Job drawing, mm, ordinate dimensions from the low corner. One solid piece. A direction names the side the tool comes from. Give positions to 0.01 mm unless a question says otherwise; leave off trailing zeros. Order: outer loops, then holes, each group sorted by start corner. A loop starts at its lowest first (then second) coordinate and runs counter-clockwise, first axis right, second up. Notation, with made-up numbers: M 79.5,65 L 100.5,65 A16 cw 100.5,70 Z; hole C -32,-28.75 d9. An arc over 180 degrees is marked long. One line per question, with ' | ' between items.
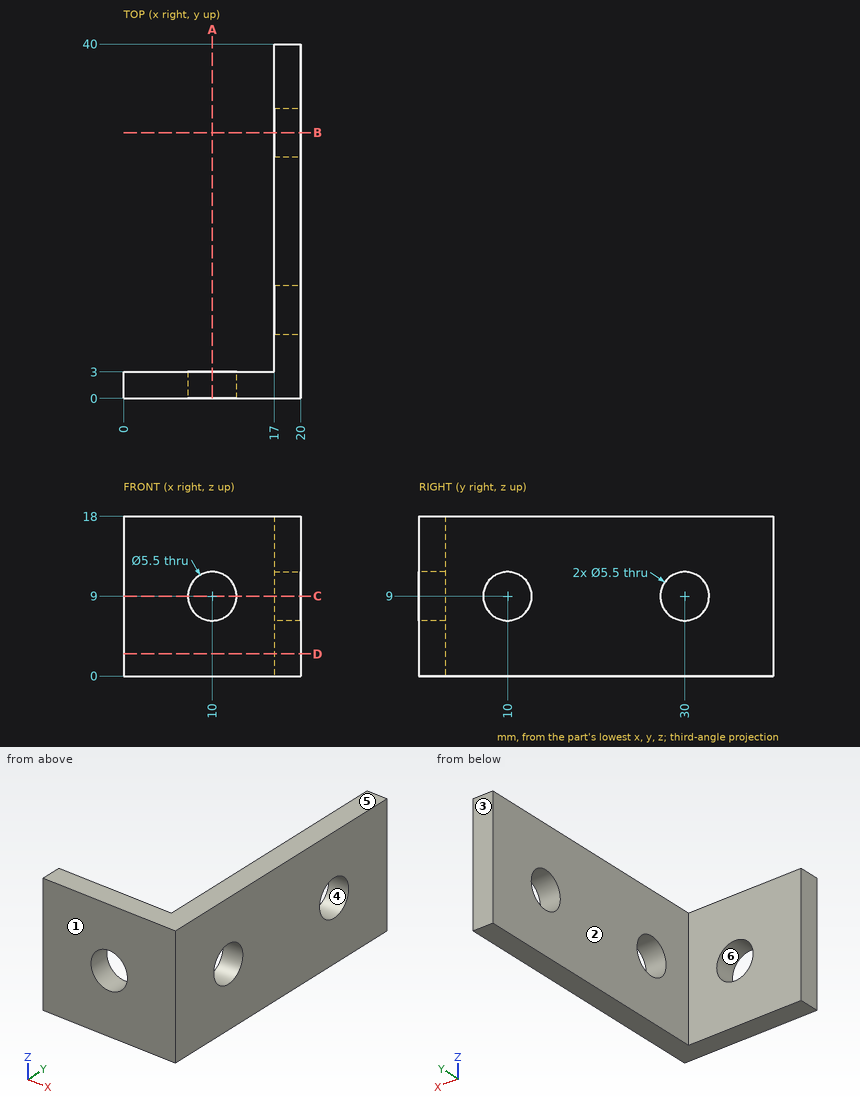
1. Slice it at C-C on z = 9. Give the cut face in (x, y), then the cut area to 4 significant figures.
Worked out:
outline: M 0,0 L 7.25,0 L 7.25,3 L 0,3 Z; M 12.75,0 L 20,0 L 20,7.25 L 17,7.25 L 17,3 L 12.75,3 Z; M 17,12.75 L 20,12.75 L 20,27.25 L 17,27.25 Z; M 17,32.75 L 20,32.75 L 20,40 L 17,40 Z | area: 121.5 mm2
2. Probe L1, parallel to Y at x = 19.4, z = 9; L2, parallel to Z at x = 10, y = 1.75; L3, parallel to Y at x = 2, z = 16.25. List the from-to ranges inside material, lowest first. Write a range as from..to.
Worked out:
L1: y = 0..7.25, 12.75..27.25, 32.75..40 | L2: z = 0..6.25, 11.75..18 | L3: y = 0..3
3. Slice it at B-B on y = 30. Give the cut face in (x, z), then the cut area to 3 significant figures.
Worked out:
outline: M 17,0 L 20,0 L 20,6.25 L 17,6.25 Z; M 17,11.75 L 20,11.75 L 20,18 L 17,18 Z | area: 37.5 mm2
4. Drop flat-ended pins along their axis: pin 1 (6 mm diameter, centred on x = 6, y = 8.5, fed in from +Z); pin 2 (7 mm diameter, centred on y = 30, z = 9, fed in from -X); pin 3 (10 mm diameter, centred on x = 6.5, z = 11.5, fed in from +Y). Give the stop position or say it passes through.
Worked out:
pin 1: passes through | pin 2: stops at x = 17 | pin 3: stops at y = 3
5. Mould opens along Z. For the marked faces 3, 4, 5 and 6 say: released by +Z, released by -Z, zero draft, split by the parting line, or undercut.
Worked out:
face 3: zero draft | face 4: undercut | face 5: released by +Z | face 6: undercut
6. Slice it at A-A on x = 10. Give the cut face in (y, z), then the cut area to 3 significant figures.
Worked out:
outline: M 0,0 L 3,0 L 3,6.25 L 0,6.25 Z; M 0,11.75 L 3,11.75 L 3,18 L 0,18 Z | area: 37.5 mm2
7. Slice it at D-D on z = 2.5. Give the cut face in (x, y), then the cut area to 3 significant figures.
Worked out:
outline: M 0,0 L 20,0 L 20,40 L 17,40 L 17,3 L 0,3 Z | area: 171 mm2
8. Tool access for the marked faces 1 and 2: list every direction of +Z, -Z, +X, -X, +Y, -Y with a clear straight run to the whole face (end or side of a thin tool).
Worked out:
face 1: +Z, -Z, +X, -X, -Y | face 2: +Z, -Z, -X, +Y
